Source: CAD feature listing. Evaluate the final solid. Frame: model axes, mm. A direction names the side the tool comes from. Coordinates: 2 decimals unless noted, no trailing zeros. Write each loop counter-clockwise with the first axis right and the second up, starting at its lowest first coordinate (ties: lowest second). Pieces come first, ordered by that corner, then holes. Notation, with made-up numbers: M 22.5,60 L 78.5,60 A31 cw 78.5,94 Z; hole C 89,-18.75 d5. An arc over 180 degrees is marked long. Answer as CSV lines item,"result". Start each with the question number.
1. Section C-C on z = -31.5. Return the cut outline in (x, y), plus the area to 3 significant figures.
2. Contact query for flat-ended pins moving along their axis: pin 1 Ø3 at (x, z) = (22.5, -14) entering from +Y; pin 2 Ø2 at (x, z) = (-20, 4) entering from -Y; pin 3 Ø12 at (x, z) = (-12.5, -22.5) entering from -Y. Output: stop coordinate, or through.
3. Mould query, pull axis X, two halves, no side actions, for faces 5 (the face through (-29.97, 1.32, -37.97)), 6 (the face through (-14, -24, -25)), 7 (the face through (6, -20, 40)). Classes: pulls with the +X half, pulls with the -X half, needs draft (parallel to the pull), parting line crosses it, or undercut.
4. Section A-A on x = 0. Count the separate pieces of the cut face and the enclosed holes in it, plus the area to 3 significant figures.
5. Line query: probe 1 along Z at (x, y) = (11.5, 24); probe 2 along X at (y, z) = (0, 22.5); probe 3 along Z at (x, y) = (-20, 11.5). Output: solid intervals per line, ascending. Write a range as [from, to].
6. Reachability of faces 1 (the face through (-23, 0, 25)), 2 (the face through (27, 0, 25)), 3 (the face through (-14, 24, 25)), 4 (the face through (-29.97, 1.32, 37.97)) from +Z, -Z, +X, -X, +Y, -Y: full face, straight path, thin tool, end or side. Return the list, or none.
```python
from build123d import *
from build123d.topology import SkipClean

# Parameters (mm, degrees)
SKETCH_1_R               = 25
SKETCH_1_R_2             = 20
EXTRUDE_1_DEPTH          = 40
EXTRUDE_START            = -15
SKETCH_2_R               = 30
SKETCH_2_R_2             = 25
EXTRUDE_2_DEPTH          = 15
EXTRUDE_START_2          = 25
EXTRUDE_3_DEPTH          = 25
PATTERN_CIRCULAR_1_COUNT = 3
CUT_EXTRUDE_1_DEPTH      = 25
PATTERN_CIRCULAR_2_COUNT = 3
SKETCH_6_R               = 0.75
CUT_EXTRUDE_2_DEPTH      = 40
PATTERN_CIRCULAR_4_COUNT = 3
CUT_EXTRUDE_3_DEPTH      = 3
CUT_EXTRUDE_3_DEPTH_BACK = 3
SKETCH_11_R              = 30
SKETCH_11_R_2            = 25
SKETCH_13_R              = 0.75
CUT_EXTRUDE_5_DEPTH      = 52.961524285
PATTERN_CIRCULAR_3_COUNT = 3


with BuildPart() as part:
    # 草图1 → 凸台-拉伸1 (new body)
    with BuildSketch(Plane.XY):
        Circle(SKETCH_1_R)
        Circle(SKETCH_1_R_2, mode=Mode.SUBTRACT)
    extrude(amount=EXTRUDE_1_DEPTH)

    # 草图2 → 凸台-拉伸2 (add)
    with BuildSketch(Plane.XY.offset(40).offset(EXTRUDE_START)):
        Circle(SKETCH_2_R)
        Circle(SKETCH_2_R_2, mode=Mode.SUBTRACT)
    extrude(amount=EXTRUDE_2_DEPTH)

    # 草图3 → 凸台-拉伸3 (add)
    with BuildSketch(Plane(origin=(0, 0, 25), x_dir=(-1, 0, 0), z_dir=(0, 0, -1)).offset(EXTRUDE_START_2)):
        with BuildLine():
            Line((-24.786121534, 3.263154806), (-29.743345841, 3.915785767))
            ThreePointArc((-29.743345841, 3.915785767), (-28.977774789, 7.764571353), (-27.716385975, 11.480502971))
            Line((-27.716385975, 11.480502971), (-23.096988313, 9.567085809))
            ThreePointArc((-23.096988313, 9.567085809), (-24.148145657, 6.470476128), (-24.786121534, 3.263154806))
        make_face()
        with BuildLine():
            Line((-29.743345841, -3.915785767), (-24.786121534, -3.263154806))
            ThreePointArc((-24.786121534, -3.263154806), (-24.148145657, -6.470476128), (-23.096988313, -9.567085809))
            Line((-23.096988313, -9.567085809), (-27.716385975, -11.480502971))
            ThreePointArc((-27.716385975, -11.480502971), (-28.977774789, -7.764571353), (-29.743345841, -3.915785767))
        make_face()
    extrude_3 = extrude(amount=-EXTRUDE_3_DEPTH)

    # 阵列(圆周)1: 凸台-拉伸3 ×3 about axis
    pattern_circular_1_axis = Axis((0, 0, 0), (0, 0, 1))
    for i in range(1, PATTERN_CIRCULAR_1_COUNT):
        add(extrude_3.rotate(pattern_circular_1_axis, i * 360 / PATTERN_CIRCULAR_1_COUNT))

    # 草图5 → 切除-拉伸1 (cut)
    with BuildSketch(Plane(origin=(0, 0, 0), x_dir=(-1, 0, 0), z_dir=(0, 0, -1))):
        with BuildLine():
            Line((-23.096988313, 9.567085809), (-18.47759065, 7.653668647))
            ThreePointArc((-18.47759065, 7.653668647), (-10, 17.320508076), (2.610523844, 19.828897227))
            Line((2.610523844, 19.828897227), (3.263154806, 24.786121534))
            ThreePointArc((3.263154806, 24.786121534), (-12.5, 21.650635095), (-23.096988313, 9.567085809))
        make_face()
    cut_extrude_1 = extrude(amount=-CUT_EXTRUDE_1_DEPTH, mode=Mode.SUBTRACT)

    # 阵列(圆周)2: 切除-拉伸1 ×3 about axis
    pattern_circular_2_axis = Axis((0, 0, 40), (0, 0, -1))
    for i in range(1, PATTERN_CIRCULAR_2_COUNT):
        add(cut_extrude_1.rotate(pattern_circular_2_axis, i * 360 / PATTERN_CIRCULAR_2_COUNT), mode=Mode.SUBTRACT)

    # 草图6 → 切除-拉伸2 (cut)
    with BuildSketch(Plane.XY.offset(40)):
        with Locations((-11.079175501, 19.189694874)):
            Circle(SKETCH_6_R)
        with Locations((22.158351002, 0)):
            Circle(SKETCH_6_R)
        with Locations((-11.079175501, -19.189694874)):
            Circle(SKETCH_6_R)
    extrude(amount=-CUT_EXTRUDE_2_DEPTH, mode=Mode.SUBTRACT)

    # 草图10 → 切除-旋转3 (revolve, cut)
    with SkipClean():  # the faces are left unmerged after this step: merging them gives an invalid solid
        with BuildSketch(Plane(origin=(0, 0, 0), x_dir=(-1, 0, 0), z_dir=(0, 0, -1))):
            with BuildLine():
                ThreePointArc((-22.908351002, 0), (-22.688681088, 0.530330086), (-22.158351002, 0.75))
                Line((-22.158351002, 0.75), (-24.988747468, 0.75))
                ThreePointArc((-24.988747468, 0.75), (-24.997186709, 0.375042204), (-25, 0))
                Line((-25, 0), (-22.908351002, 0))
            make_face()
            with BuildLine():
                Line((-22.158351002, 0), (-22.158351002, 0.75))
                ThreePointArc((-22.158351002, 0.75), (-22.688681088, 0.530330086), (-22.908351002, 0))
                Line((-22.908351002, 0), (-22.158351002, 0))
            make_face()
            with BuildLine():
                Line((-22.158351002, -0.75), (-22.158351002, 0))
                Line((-22.158351002, 0), (-22.908351002, 0))
                ThreePointArc((-22.908351002, 0), (-22.688681088, -0.530330086), (-22.158351002, -0.75))
            make_face()
            with BuildLine():
                ThreePointArc((-25, 0), (-24.997186709, 0.375042204), (-24.988747468, 0.75))
                Line((-24.988747468, 0.75), (-26.146421449, 0.75))
                Line((-26.146421449, 0.75), (-26.146421449, 0))
                Line((-26.146421449, 0), (-25, 0))
            make_face()
        cut_revolve_3 = revolve(axis=Axis((22.158351002, 0, 0), (1, 0, 0)), mode=Mode.SUBTRACT)
    add(part.part.scale(1), mode=Mode.REPLACE)  # the faces are merged on a copy

    # 阵列(圆周)4: 切除-旋转3 ×3 about axis
    pattern_circular_4_axis = Axis((0, 0, 40), (0, 0, -1))
    for i in range(1, PATTERN_CIRCULAR_4_COUNT):
        add(cut_revolve_3.rotate(pattern_circular_4_axis, i * 360 / PATTERN_CIRCULAR_4_COUNT), mode=Mode.SUBTRACT)

    # 草图11 → 切除-拉伸3 (cut, two sides: drawn at the far end of the back side and taken through both)
    with BuildSketch(Plane.XY.offset(33).offset(-CUT_EXTRUDE_3_DEPTH_BACK)):
        Circle(SKETCH_11_R)
        Circle(SKETCH_11_R_2, mode=Mode.SUBTRACT)
    extrude(amount=CUT_EXTRUDE_3_DEPTH + CUT_EXTRUDE_3_DEPTH_BACK, mode=Mode.SUBTRACT)

    # 草图13 → 切除-拉伸5 (cut, through all)
    with BuildSketch(Plane.XY.offset(30)):
        with Locations((-6.998313063, 26.118059917)):
            Circle(SKETCH_13_R)
    cut_extrude_5 = extrude(amount=-CUT_EXTRUDE_5_DEPTH, mode=Mode.SUBTRACT)

    # 阵列(圆周)3: 切除-拉伸5 ×3 about axis
    pattern_circular_3_axis = Axis((0, 0, 0), (0, 0, 1))
    for i in range(1, PATTERN_CIRCULAR_3_COUNT):
        add(cut_extrude_5.rotate(pattern_circular_3_axis, i * 360 / PATTERN_CIRCULAR_3_COUNT), mode=Mode.SUBTRACT)

    # 镜向1: part across face


with BuildPart() as part_1:
    add(part.part)
    add(part.part.mirror(Plane(origin=(-11.959573357, -20.875780488, 0), x_dir=(1, 0, 0), z_dir=(0, 0, -1))))


solid = part_1.part
```
Values:
1,outline,"C 0,0 d50; hole C 0,0 d40; hole C -11.08,-19.19 d1.5; hole C -11.08,19.19 d1.5; hole C 22.16,0 d1.5"
1,area,"702 mm²"
2,pin 1,"y = 9.94"
2,pin 2,"y = -23.22"
2,pin 3,"y = -29.29"
3,face 5,"parting line crosses it"
3,face 6,"undercut"
3,face 7,"needs draft"
4,separate pieces,"4"
4,enclosed holes,"0"
4,area,"480 mm²"
5,probe 1,"[-40, -36], [-30, -25], [25, 30], [36, 40]"
5,probe 2,"[20, 21.41], [22.91, 25]"
5,probe 3,"[-40, -25], [25, 40]"
6,face 1,"-X"
6,face 2,"+X"
6,face 3,"none"
6,face 4,"+Z, -Z"
